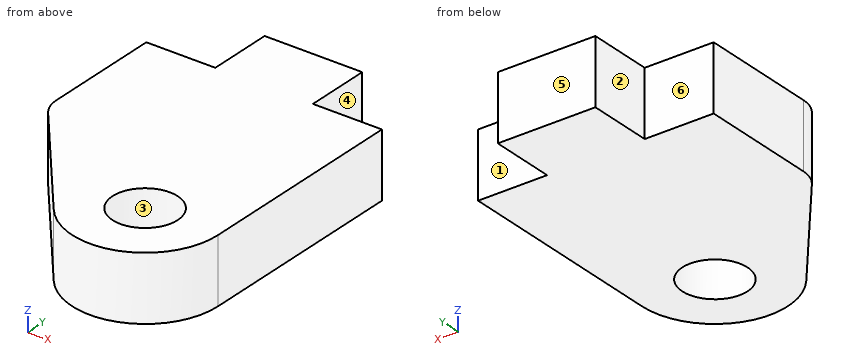
```python
from build123d import *

# Parameters (mm, degrees)
SKETCH1_R           = 1.5875
BOSS_EXTRUDE1_DEPTH = 1.5875


with BuildPart() as part:
    # Sketch1 → Boss-Extrude1 (new body, symmetric)
    with BuildSketch(Plane.XY):
        with BuildLine():
            Line((-5.74675, 0), (-5.74675, -5.791392014))
            ThreePointArc((-5.74675, -5.791392014), (-5.65674567, -6.318329362), (-5.396938386, -6.785516609))
            Line((-5.396938386, -6.785516609), (-0.581671984, -12.780539093))
            ThreePointArc((-0.581671984, -12.780539093), (3.37108966, -13.9080903), (5.74675, -10.5537))
            Line((5.74675, -10.5537), (5.74675, 0))
            Line((5.74675, 0), (2.38125, 0))
            Line((2.38125, 0), (2.38125, 3.175))
            Line((2.38125, 3.175), (-2.38125, 3.175))
            Line((-2.38125, 3.175), (-2.38125, 0))
            Line((-2.38125, 0), (-5.74675, 0))
        make_face()
        with Locations((2.19075, -10.5537)):
            Circle(SKETCH1_R, mode=Mode.SUBTRACT)
    extrude(amount=BOSS_EXTRUDE1_DEPTH, both=True)


solid = part.part
```
The listing builds one solid part. Answer for the finished solid, in the listing's coordinates (mm). Face numbers are marked on the shaded views. A direction names the side the tool comes from. Round coordinates to 2 decimals unless told otherwise and drop trailing zeros. Loops run counter-clockwise (first coordinate to the right, second up) from the corner with the lowest first, then second, coordinate; pieces in that order, holes last.
Q1. Find the intervals of material crossed by line 1 (Y direction, x = 2.25, z = -0.95) (3 decimals); line 2 (X direction, y = 2.25, z = 1.05); line 3 (X direction, y = -11, z = 0.5), in increasing order.
Q2. Given pin 1 Ø1.6 at (y, z) = (1.5, 0) entering from -X; pin 2 Ø1 at (y, z) = (1.5, 1) entering from +X; pin 3 Ø1.6 at (x, z) = (-3.5, 0.5) entering from +Y; pin 4 Ø3 at (x, y) = (2.19, -10.55) entering from +Z, each flat-ended and moving along its own axis, determine where each tip first touches the part or whether it passes through.
Q3. Section B-B, the plane y = -9.25 is taken. Determine the outline of the cut face in (x, z).
Q4. Section C-C, the plane x = 1.75 is taken. Determine the outline of the cut face in (y, z) (1 decimal), then the cut area to 3 significant figures.
Q5. For a pull along Y with two mould halves and no side action, classify the marked faces 1, 2 and 3 as released by +Y, released by -Y, zero draft, split by the parting line, or undercut.
Q6. Which of the six approach directions +Z, -Z, +X, -X, +Y, -Y give full straight-line access (tool end or side, diameter ignored) to the marked faces 4, 5 and 6?
Q7. Section D-D, the plane y = 1.25 is taken. Determine the outline of the cut face in (x, z).
Q8. Section A-A, the plane z = 0.4 is taken. Determine the outline of the cut face in (x, y) (1 decimal), then the cut area to 3 significant figures.
Completed:
1. line 1: y = -14.109 to -12.14, -8.967 to 3.175
1. line 2: x = -2.38 to 2.38
1. line 3: x = -2.01 to 0.67, 3.71 to 5.72
2. pin 1: stops at x = -2.38
2. pin 2: stops at x = 2.38
2. pin 3: stops at y = 0
2. pin 4: passes through
3. outline: (-3.42, -1.59) - (1.28, -1.59) - (1.28, 1.59) - (-3.42, 1.59) - close; (3.1, -1.59) - (5.75, -1.59) - (5.75, 1.59) - (3.1, 1.59) - close
4. outline: (-14.1, -1.6) - (-12.1, -1.6) - (-12.1, 1.6) - (-14.1, 1.6) - close; (-9, -1.6) - (3.2, -1.6) - (3.2, 1.6) - (-9, 1.6) - close
4. area: 45.1 mm2
5. face 1: released by +Y
5. face 2: zero draft
5. face 3: undercut
6. face 4: +Z, -Z, +X, +Y
6. face 5: +Z, -Z, +X, -X, +Y
6. face 6: +Z, -Z, -X, +Y
7. outline: (-2.38, -1.59) - (2.38, -1.59) - (2.38, 1.59) - (-2.38, 1.59) - close
8. outline: (-5.7, -5.8) arc R1.6 ccw to (-5.4, -6.8) - (-0.6, -12.8) arc R3.6 ccw to (5.7, -10.6) - (5.7, 0) - (2.4, 0) - (2.4, 3.2) - (-2.4, 3.2) - (-2.4, 0) - (-5.7, 0) - close; hole circle Ø3.2 at (2.2, -10.6)
8. area: 142 mm2
